Here's how the part is built. I have some questions about the finished solid (model axes, mm). Face numbers are marked on the shaded views. A direction names the side the tool comes from. Coordinates: 2 decimals unless noted, no trailing zeros. Write each loop counter-clockwise with the first axis right and the second up, starting at its lowest first coordinate (ties: lowest second). Pieces come first, ordered by that corner, then holes.
(1) Which directions (+Z, -Z, +X, -X, +Y, -Y) give clear straight access to the entire face, cutting with the end or side of a thin tool? Please do the marked faces 1, 2 and 3.
(2) Thinking about a two-plate mould opening in X: for the marked faces 4, 5, 6 and 7, which applies, released by +X, released by -X, zero draft, split by the parting line, or undercut?
(3) Imagine slicing it at A-A, the plane x = 13. List the corners of the cut face in (y, z) for me (1 decimal).
(4) Imagine slicing it at C-C, the plane x = 25.4. State how many separate pieces and enclosed holes the cut face has, plus the area to 3 significant figures.
(5) For pin 1 Ø8 at (x, z) = (98.5, -44) entering from -Y; pin 2 Ø12 at (x, z) = (86, -27) entering from -Y, each with a flat end and sliding along its axis, tell me the tip position at first contact or that it passes through.
(6) Imagine slicing it at B-B, the plane z = -46. List the corners of the cut face in (x, y) for me.
(7) Imagine slicing it at D-D, the plane y = -5.75. List the corners of the cut face in (x, z) for me (1 decimal), plus the area to 3 significant figures.
(8) Please list where these lines run through material, in increasing order: probe 1 along Z at (x, y) = (74, 2) (1 decimal); probe 2 along X at (y, z) = (-2.25, -56); probe 3 along Z at (x, y) = (63.5, 0.75) (1 decimal).
```python
from build123d import *

# Parameters (mm, degrees)
SKETCH1_W                    = 104.687624
SKETCH1_H                    = 60.325
SKETCH1_W_2                  = 35.675062
SKETCH1_H_2                  = 38.1
BOSS_EXTRUDE1_DEPTH          = 11.1125
BOSS_EXTRUDE32_DEPTH         = 11.1125
BOSS_EXTRUDE36_START         = -49.2125
BOSS_EXTRUDE36_DEPTH         = 11.1125
CUT_EXTRUDE1_REACH           = 22.637
SKETCH9_W                    = 11.1125
SKETCH9_H                    = 12.7
BOSS_EXTRUDE37_REACH         = 38.512
SKETCH10_R                   = 3.175
F_97_0_0059_DIAMETER_HOLE1_D = 6.35
SKETCH17_R                   = 3.556
CUT_EXTRUDE2_DEPTH           = 1.778
SKETCH18_R                   = 3.556
CUT_EXTRUDE3_DEPTH           = 1.778
SKETCH19_R                   = 3.175
CUT_EXTRUDE4_DEPTH           = 5.842
SKETCH20_R                   = 3.556
CUT_EXTRUDE7_DEPTH           = 6.842
CUT_EXTRUDE7_DEPTH_BACK      = 15.7955
SKETCH24_R                   = 3.556
SKETCH24_R_2                 = 3.175
BOSS_EXTRUDE40_DEPTH         = 5.842


with BuildPart() as part:
    # Sketch1 → Boss-Extrude1 (new body)
    with BuildSketch(Plane(origin=(0, 0, 0), x_dir=(1, 0, 0), z_dir=(0, 1, 0))):
        with Locations((52.343812, 30.1625)):
            Rectangle(SKETCH1_W, SKETCH1_H)
        with Locations((28.950031, 30.1625)):
            Rectangle(SKETCH1_W_2, SKETCH1_H_2, mode=Mode.SUBTRACT)
        with Locations((75.737593, 30.1625)):
            Rectangle(SKETCH1_W_2, SKETCH1_H_2, mode=Mode.SUBTRACT)
    extrude(amount=BOSS_EXTRUDE1_DEPTH)

    # Sketch2 → Boss-Extrude32 (add)
    with BuildSketch(Plane.XY):
        with BuildLine():
            Line((0, 11.1125), (0, 0))
            Line((0, 0), (15.875, 0))
            ThreePointArc((15.875, 0), (25.4, -9.525), (34.925, 0))
            Line((34.925, 0), (69.762624, 0))
            ThreePointArc((69.762624, 0), (79.287624, -9.525), (88.812624, 0))
            Line((88.812624, 0), (104.687624, 0))
            Line((104.687624, 0), (104.687624, 11.1125))
            Line((104.687624, 11.1125), (0, 11.1125))
        make_face()
    extrude(amount=-BOSS_EXTRUDE32_DEPTH)

    # Sketch2<11> → Boss-Extrude36 (add)
    with BuildSketch(Plane.XY.offset(BOSS_EXTRUDE36_START)):
        with BuildLine():
            Line((0, 11.1125), (0, 0))
            Line((0, 0), (15.875, 0))
            ThreePointArc((15.875, 0), (25.4, -9.525), (34.925, 0))
            Line((34.925, 0), (69.762624, 0))
            ThreePointArc((69.762624, 0), (79.287624, -9.525), (88.812624, 0))
            Line((88.812624, 0), (104.687624, 0))
            Line((104.687624, 0), (104.687624, 11.1125))
            Line((104.687624, 11.1125), (0, 11.1125))
        make_face()
    extrude(amount=-BOSS_EXTRUDE36_DEPTH)

    # Sketch9 → Cut-Extrude1 (cut, up to next)
    with BuildSketch(Plane(origin=(0, 11.1125, 0), x_dir=(1, 0, 0), z_dir=(0, 1, 0)), mode=Mode.PRIVATE) as cut_extrude1_sk1:
        with Locations((99.131374, 30.1625)):
            Rectangle(SKETCH9_W, SKETCH9_H)
    cut_extrude1_tool1 = extrude(cut_extrude1_sk1.sketch, amount=-CUT_EXTRUDE1_REACH, mode=Mode.PRIVATE) & part.part
    add(cut_extrude1_tool1.solids().sort_by_distance((99.131374, 11.1125, -30.1625))[0], mode=Mode.SUBTRACT)

    # Sketch10 → Boss-Extrude37 (add, up to next)
    with BuildSketch(Plane.XY.offset(-36.5125), mode=Mode.PRIVATE) as boss_extrude37_sk1:
        with Locations((99.131374, 7.9375)):
            Circle(SKETCH10_R)
    boss_extrude37_tool1 = extrude(boss_extrude37_sk1.sketch, amount=BOSS_EXTRUDE37_REACH, mode=Mode.PRIVATE) - part.part
    add(boss_extrude37_tool1.solids().sort_by_distance((99.131374, 7.9375, -36.5125))[0])

    # #97 (0.0059) Diameter Hole1 (through all)
    with Locations(Plane.XY):
        with Locations((25.4, 0), (79.287624, 0)):
            Hole(F_97_0_0059_DIAMETER_HOLE1_D / 2)

    # Sketch17 → Cut-Extrude2 (cut)
    with BuildSketch(Plane(origin=(0, 0, -11.1125), x_dir=(-1, 0, 0), z_dir=(0, 0, -1))):
        with Locations((-25.4, 0)):
            Circle(SKETCH17_R)
        with Locations((-79.287624, 0)):
            Circle(SKETCH17_R)
    extrude(amount=-CUT_EXTRUDE2_DEPTH, mode=Mode.SUBTRACT)

    # Sketch18 → Cut-Extrude3 (cut)
    with BuildSketch(Plane.XY.offset(-49.2125)):
        with Locations((25.4, 0)):
            Circle(SKETCH18_R)
        with Locations((79.287624, 0)):
            Circle(SKETCH18_R)
    extrude(amount=-CUT_EXTRUDE3_DEPTH, mode=Mode.SUBTRACT)

    # Sketch19 → Cut-Extrude4 (cut)
    with BuildSketch(Plane(origin=(0, 11.1125, 0), x_dir=(1, 0, 0), z_dir=(0, 1, 0))):
        with Locations((99.036124, 54.76875)):
            Circle(SKETCH19_R)
        with Locations((64.487044, 54.76875)):
            Circle(SKETCH19_R)
        with Locations((-40.811196, 54.76875)):
            Circle(SKETCH19_R)
        with Locations((99.036124, 5.55625)):
            Circle(SKETCH19_R)
        with Locations((64.487044, 5.55625)):
            Circle(SKETCH19_R)
        with Locations((-40.811196, 5.55625)):
            Circle(SKETCH19_R)
    extrude(amount=-CUT_EXTRUDE4_DEPTH, mode=Mode.SUBTRACT)

    # Sketch20 → Cut-Extrude7 (cut, two sides)
    with BuildSketch(Plane(origin=(0, 5.2705, 0), x_dir=(1, 0, 0), z_dir=(0, 1, 0))) as cut_extrude7_sk:
        with Locations((99.036124, 54.76875)):
            Circle(SKETCH20_R)
        with Locations((64.487044, 54.76875)):
            Circle(SKETCH20_R)
        with Locations((6.90118, 54.76875)):
            Circle(SKETCH20_R)
        with Locations((6.90118, 5.55625)):
            Circle(SKETCH20_R)
        with Locations((64.487044, 5.55625)):
            Circle(SKETCH20_R)
        with Locations((99.036124, 5.55625)):
            Circle(SKETCH20_R)
    extrude(amount=CUT_EXTRUDE7_DEPTH, mode=Mode.SUBTRACT)
    extrude(cut_extrude7_sk.sketch, amount=-CUT_EXTRUDE7_DEPTH_BACK, mode=Mode.SUBTRACT)

    # Sketch24 → Boss-Extrude40 (add)
    with BuildSketch(Plane(origin=(0, 11.1125, 0), x_dir=(1, 0, 0), z_dir=(0, 1, 0))):
        with Locations((64.487044, 5.55625)):
            Circle(SKETCH24_R)
        with Locations((64.487044, 5.55625)):
            Circle(SKETCH24_R_2, mode=Mode.SUBTRACT)
        with Locations((6.90118, 54.76875)):
            Circle(SKETCH24_R)
        with Locations((6.90118, 54.76875)):
            Circle(SKETCH24_R_2, mode=Mode.SUBTRACT)
        with Locations((64.487044, 54.76875)):
            Circle(SKETCH24_R)
        with Locations((64.487044, 54.76875)):
            Circle(SKETCH24_R_2, mode=Mode.SUBTRACT)
        with Locations((99.036124, 54.76875)):
            Circle(SKETCH24_R)
        with Locations((99.036124, 54.76875)):
            Circle(SKETCH24_R_2, mode=Mode.SUBTRACT)
        with Locations((99.036124, 5.55625)):
            Circle(SKETCH24_R)
        with Locations((99.036124, 5.55625)):
            Circle(SKETCH24_R_2, mode=Mode.SUBTRACT)
        with Locations((6.90118, 5.55625)):
            Circle(SKETCH24_R)
        with Locations((6.90118, 5.55625)):
            Circle(SKETCH24_R_2, mode=Mode.SUBTRACT)
    extrude(amount=-BOSS_EXTRUDE40_DEPTH)


solid = part.part
```
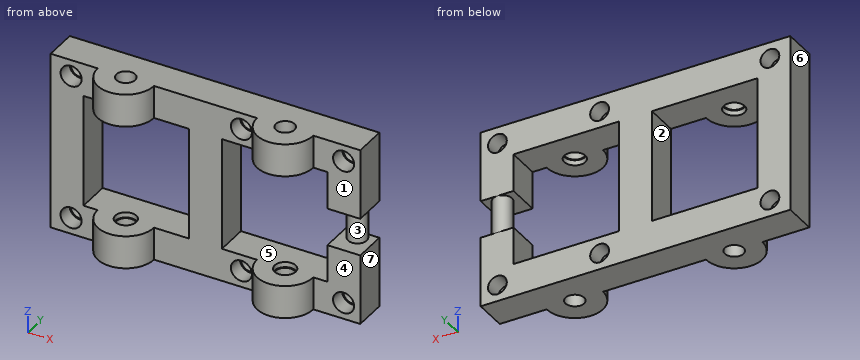
Recorded:
1. face 1: +Z, -Z, +X, -Y
1. face 2: +Y, -Y
1. face 3: none
2. face 4: zero draft
2. face 5: undercut
2. face 6: released by -X
2. face 7: released by +X
3. outline: (0, -60.3) - (11.1, -60.3) - (11.1, -49.2) - (0, -49.2) - close; (0, -11.1) - (11.1, -11.1) - (11.1, 0) - (0, 0) - close
4. separate pieces: 4
4. enclosed holes: 0
4. area: 315 mm2
5. pin 1: stops at y = 0
5. pin 2: passes through
6. outline: (0, 0) - (11.11, 0) - (11.11, 11.11) - (0, 11.11) - close; (46.79, 0) - (57.9, 0) - (57.9, 11.11) - (46.79, 11.11) - close; (93.58, 0) - (104.69, 0) - (104.69, 11.11) - (93.58, 11.11) - close
7. outline: (17.8, -60.3) - (33, -60.3) - (33, -49.2) - (17.8, -49.2) - close; (17.8, -11.1) - (33, -11.1) - (33, 0) - (17.8, 0) - close; (71.7, -60.3) - (86.9, -60.3) - (86.9, -49.2) - (71.7, -49.2) - close; (71.7, -11.1) - (86.9, -11.1) - (86.9, 0) - (71.7, 0) - close
7. area: 675 mm2
8. probe 1: z = -60.3 to -49.2, -11.1 to 0
8. probe 2: x = 16.14 to 23.16, 27.64 to 34.66, 70.03 to 77.05, 81.53 to 88.54
8. probe 3: z = -60.3 to -58.2, -51.4 to -49.2, -11.1 to -9, -2.1 to 0
